```python
from build123d import *

# Parameters (mm, degrees)
SKETCH_W        = 71
SKETCH_H        = 76
PAD_DEPTH       = 49
SKETCH001_W     = 67
SKETCH001_H     = 72
POCKET_DEPTH    = 47
SKETCH002_W     = 14
SKETCH002_H     = 22
POCKET001_DEPTH = 2
SKETCH003_R     = 4
SKETCH003_W     = 36
SKETCH003_H     = 6
POCKET002_DEPTH = 49.001
CHAMFER_SIZE    = 1
POCKET003_DEPTH = 49.001
CHAMFER001_SIZE = 0.5


with BuildPart() as part:
    # Sketch → Pad (new body)
    with BuildSketch(Plane.XY):
        Rectangle(SKETCH_W, SKETCH_H)
    extrude(amount=PAD_DEPTH)

    # Sketch001 (on Face5 of Pad) → Pocket (cut)
    with BuildSketch(Plane(origin=(0, 0, 0), x_dir=(1, 0, 0), z_dir=(0, 0, -1))):
        Rectangle(SKETCH001_W, SKETCH001_H)
    extrude(amount=-POCKET_DEPTH, mode=Mode.SUBTRACT)

    # Sketch002 (on Face6 of Pocket) → Pocket001 (cut)
    with BuildSketch(Plane.XZ.offset(38)):
        with Locations((-23.5, 11)):
            Rectangle(SKETCH002_W, SKETCH002_H)
    extrude(amount=-POCKET001_DEPTH, mode=Mode.SUBTRACT)

    # Sketch003 (on Face4 of Pocket001) → Pocket002 (cut, through all)
    with BuildSketch(Plane.XY.offset(49)):
        with Locations((0, 24)):
            Circle(SKETCH003_R)
        with Locations((-8.5, -19)):
            Rectangle(SKETCH003_W, SKETCH003_H)
        with BuildLine():
            Line((26.5, -23.5), (17.5, -23.5))
            Line((17.5, -23.5), (17.5, -21.872281))
            ThreePointArc((17.5, -16.127719), (12, -19), (17.5, -21.872281))
            Line((17.5, -14.5), (17.5, -16.127719))
            Line((17.5, -14.5), (26.5, -14.5))
            Line((26.5, -14.5), (26.5, -23.5))
        make_face()
    extrude(amount=-POCKET002_DEPTH, mode=Mode.SUBTRACT)

    # Chamfer
    chamfer_edges = [part.edges().sort_by_distance(p)[0] for p in [
        (22, -23.5, 49),
        (12, -19, 49),
        (17.5, -22.686141, 49),
        (17.5, -15.313859, 49),
        (22, -14.5, 49),
        (26.5, -19, 49),
        (9.5, -19, 49),
        (-8.5, -22, 49),
        (-8.5, -16, 49),
        (-26.5, -19, 49),
        (0, 38, 49),
        (35.5, 0, 49),
        (0, -38, 49),
        (-35.5, 0, 49),
        (0, -36, 47),
        (33.5, 0, 47),
        (-33.5, 0, 47),
        (0, 36, 47),
        (-35.5, -38, 24.5),
        (-35.5, 38, 24.5),
        (35.5, -38, 24.5),
        (35.5, 38, 24.5),
        (33.5, -36, 23.5),
        (33.5, 36, 23.5),
        (-33.5, 36, 23.5),
        (-33.5, -36, 23.5),
        (-23.5, -38, 22),
        (-30.5, -38, 11),
        (-16.5, -38, 11),
    ]]
    chamfer(chamfer_edges, length=CHAMFER_SIZE)

    # Sketch004 (on Face25 of Chamfer) → Pocket003 (cut, through all)
    with BuildSketch(Plane.XY.offset(49)):
        with BuildLine():
            ThreePointArc((-20, 10), (-21.5, 8.5), (-20, 7))
            Line((-20, 7), (20, 7))
            ThreePointArc((20, 7), (21.5, 8.5), (20, 10))
            Line((-20, 10), (20, 10))
        make_face()
        with BuildLine():
            ThreePointArc((-20, 4), (-21.5, 2.5), (-20, 1))
            Line((-20, 1), (20, 1))
            ThreePointArc((20, 1), (21.5, 2.5), (20, 4))
            Line((-20, 4), (20, 4))
        make_face()
        with BuildLine():
            ThreePointArc((-20, -2), (-21.5, -3.5), (-20, -5))
            Line((-20, -5), (20, -5))
            ThreePointArc((20, -5), (21.5, -3.5), (20, -2))
            Line((-20, -2), (20, -2))
        make_face()
    extrude(amount=-POCKET003_DEPTH, mode=Mode.SUBTRACT)

    # Chamfer001
    chamfer001_edges = [part.edges().sort_by_distance(p)[0] for p in [
        (0, -5, 49),
        (0, 1, 49),
        (0, 7, 49),
    ]]
    chamfer(chamfer001_edges, length=CHAMFER001_SIZE)


solid = part.part
```
Here's how the part is built. I have some questions about the finished solid (model axes, mm). A direction names the side the tool comes from. Give positions to 0.01 mm unless a question says otherwise; leave off trailing zeros. Write each loop counter-clockwise with the first axis right and the second up, starting at its lowest first coordinate (ties: lowest second). Pieces come first, ordered by that corner, then holes. Notation, with made-up numbers: M 4,-14 L 60,-14 A18 cw 60,8 Z; hole C 8,74.5 d7. An arc over 180 degrees is marked long. Put each result on its own line as item: value. Start each with the question number.
Item 1: If we section it at A-A, the plane y = -19: Write out the boundary of the cut face in (x, z), then the cut area to 3 significant figures.
Item 2: If we section it at D-D, the plane x = 0: Count the separate pieces of the cut face and the enclosed holes in it, then the cut area to 3 significant figures.
Item 3: If we section it at B-B, the plane y = 24: Write out the boundary of the cut face in (x, z).
Item 4: Thinking about a two-plate mould opening in Y: for faces 1 (the flat face through (7, -38, 24)), 2 (the conical face through (21.635, 8.464, 48.635)), 3 (the flat face through (0, -8, 49)), 4 (the flat face through (0, 38, 24)), which applies, +Y half, -Y half, draft (parallel to the pull), parting line (faces both ways), or undercut?
Item 5: On a 3-axis mill with a long thin cutter (end or side, diameter ignored), from which of +Z, -Z, +X, -X, +Y, -Y can I reach the whole of each face in a straight line? I mean faces 5 (the flat face through (-35.5, -1, 24)), 6 (the flat face through (0, 36, 23)), 7 (the conical face through (21.635, 2.464, 48.635)). Say none if no direction works.
Item 6: If we section it at C-C, the plane z = 35: Write out the boundary of the cut face in (x, y).
Item 7: I need wall thicknesses on L1, parallel to X at y = -19, z = 47.75; L2, parallel to X at y = -6.5, z = 11; L3, parallel to Y at x = 15.5, z = 47.35. Which ranges of each line are inside material? Lowest first, please. Write a range as from..to.
Item 8: Will these pins go through, and if not, where does the flat tip stop? pin 1 (3 mm diameter, centred on x = -12.5, y = 13, fed in from -Z); pin 2 (1.1 mm diameter, centred on x = -21, y = -36.5, fed in from -Z); pin 3 (1.5 mm diameter, centred on x = 3, y = -16, fed in from +Z); pin 4 (6.5 mm diameter, centred on x = 0, y = 24, fed in from -Z).
Values:
1. outline: M -35.5,0 L -33.5,0 L -33.5,46 L -32.5,47 L -26.5,47 L -26.5,48 L -27.5,49 L -34.5,49 L -35.5,48 Z; M 9.5,47 L 12,47 L 12,48 L 11,49 L 10.5,49 L 9.5,48 Z; M 26.5,47 L 32.5,47 L 33.5,46 L 33.5,0 L 35.5,0 L 35.5,48 L 34.5,49 L 27.5,49 L 26.5,48 Z
1. area: 227 mm²
2. separate pieces: 6
2. enclosed holes: 0
2. area: 292 mm²
3. outline: M -35.5,0 L -33.5,0 L -33.5,46 L -32.5,47 L -4,47 L -4,49 L -34.5,49 L -35.5,48 Z; M 4,47 L 32.5,47 L 33.5,46 L 33.5,0 L 35.5,0 L 35.5,48 L 34.5,49 L 4,49 Z
4. face 1: -Y half
4. face 2: undercut
4. face 3: draft
4. face 4: +Y half
5. face 5: +Z, -Z, -X, +Y, -Y
5. face 6: -Z
5. face 7: +Z
6. outline: M -35.5,-37 L -34.5,-38 L 34.5,-38 L 35.5,-37 L 35.5,37 L 34.5,38 L -34.5,38 L -35.5,37 Z; hole M -33.5,-35 L -32.5,-36 L 32.5,-36 L 33.5,-35 L 33.5,35 L 32.5,36 L -32.5,36 L -33.5,35 Z
7. L1: -35.5..-26.5, 9.5..12, 26.5..35.5
7. L2: -35.5..-33.5, 33.5..35.5
7. L3: -38..-22.5, -15.5..-5, -2..1, 4..7, 10..38
8. pin 1: z = 47
8. pin 2: z = 22
8. pin 3: z = 48.75
8. pin 4: through
